```python
from build123d import *

# Parameters (mm, degrees)
F1_DEPTH  = 2
F2_R      = 2.5
F3_DEPTH  = 1.5
F4_R      = 1.3
F5_DEPTH  = 1.5
F7_DEPTH  = 7
F8_R      = 1.5
F9_DEPTH  = 10
F10_W     = 12.6
F10_H     = 2
F10_W_2   = 9.5
F11_DEPTH = 3.8
F12_R     = 3
F13_DEPTH = 0.4
F14_SIZE  = 1.49999
F15_W     = 19.2
F15_H     = 1.1
F16_DEPTH = 1


# Not quite as in the source:
# - a fillet or chamfer is up to 0.001 mm smaller than in the source, because OpenCascade refuses the exact size


with BuildPart() as f1:
    # F0 (on Top) → F1 (new body)
    with BuildSketch(Plane.XY):
        with BuildLine():
            Line((27.5, 38.5), (-27.5, 38.5))
            ThreePointArc((-27.5, 38.5), (-33.8639610307, 35.8639610307), (-36.5, 29.5))
            Line((-36.5, 29.5), (-36.5, -27.5))
            ThreePointArc((-36.5, -27.5), (-33.8639610307, -33.8639610307), (-27.5, -36.5))
            Line((-27.5, -36.5), (27.5, -36.5))
            ThreePointArc((27.5, -36.5), (33.8639610307, -33.8639610307), (36.5, -27.5))
            Line((36.5, -27.5), (36.5, 29.5))
            ThreePointArc((36.5, 29.5), (33.8639610307, 35.8639610307), (27.5, 38.5))
        make_face()
    extrude(amount=F1_DEPTH)

    # F2 (on face) → F3 (join)
    with BuildSketch(Plane.XY.offset(2)):
        with Locations((-19.24, -30.6)):
            Circle(F2_R)
        with Locations((8.96, -30.6)):
            Circle(F2_R)
        with Locations((24.16, 20.2)):
            Circle(F2_R)
        with Locations((-24.24, 21.5)):
            Circle(F2_R)
    extrude(amount=F3_DEPTH)

    # F4 (on face) → F5 (join)
    with BuildSketch(Plane.XY.offset(3.5)):
        with Locations((-19.24, -30.6)):
            Circle(F4_R)
        with Locations((8.96, -30.6)):
            Circle(F4_R)
        with Locations((24.16, 20.2)):
            Circle(F4_R)
        with Locations((-24.24, 21.5)):
            Circle(F4_R)
    extrude(amount=F5_DEPTH)

    # F6 (on face) → F7 (join)
    with BuildSketch(Plane.XY.offset(2)):
        with BuildLine():
            Line((27.5, 38.5), (-27.5, 38.5))
            ThreePointArc((-27.5, 38.5), (-33.8639610307, 35.8639610307), (-36.5, 29.5))
            Line((-36.5, 29.5), (-36.5, -27.5))
            ThreePointArc((-36.5, -27.5), (-33.8639610307, -33.8639610307), (-27.5, -36.5))
            Line((-27.5, -36.5), (27.5, -36.5))
            ThreePointArc((27.5, -36.5), (33.8639610307, -33.8639610307), (36.5, -27.5))
            Line((36.5, -27.5), (36.5, 29.5))
            ThreePointArc((36.5, 29.5), (33.8639610307, 35.8639610307), (27.5, 38.5))
        make_face()
        Polygon((-27.5, 29.5), (-27.5, 36.5), (27.5, 36.5), (27.5, 29.5), (34.5, 29.5), (34.5, -27.5), (27.5, -27.5), (27.5, -34.5), (-27.5, -34.5), (-27.5, -27.5), (-34.5, -27.5), (-34.5, 29.5), align=None, mode=Mode.SUBTRACT)
    extrude(amount=F7_DEPTH)

    # F8 (on face) → F9 (cut)
    with BuildSketch(Plane.XY.offset(9)):
        with Locations((-31, 33)):
            Circle(F8_R)
        with Locations((31, 33)):
            Circle(F8_R)
        with Locations((-31, -31)):
            Circle(F8_R)
        with Locations((31, -31)):
            Circle(F8_R)
    extrude(amount=-F9_DEPTH, mode=Mode.SUBTRACT)

    # F10 (on face) → F11 (cut)
    with BuildSketch(Plane.XY.offset(9)):
        with Locations((11.36, 37.5)):
            Rectangle(F10_W, F10_H)
        with Locations((-18.89, 37.5)):
            Rectangle(F10_W_2, F10_H)
    extrude(amount=-F11_DEPTH, mode=Mode.SUBTRACT)

    # F12 (on face) → F13 (cut)
    with BuildSketch(Plane(origin=(0, 0, 0), x_dir=(1, 0, 0), z_dir=(0, 0, -1))):
        with Locations((31, -33)):
            Circle(F12_R)
        with Locations((-31, -33)):
            Circle(F12_R)
        with Locations((-31, 31)):
            Circle(F12_R)
        with Locations((31, 31)):
            Circle(F12_R)
    extrude(amount=-F13_DEPTH, mode=Mode.SUBTRACT)

    # F14 (size 1.5 in the source; OpenCascade refuses exactly that, so slightly less here)
    f14_edges = [f1.edges().sort_by_distance(p)[0] for p in [
        (29.5, 33, 0.4),
        (-32.5, 33, 0.4),
        (29.5, -31, 0.4),
        (-32.5, -31, 0.4),
    ]]
    chamfer(f14_edges, length=F14_SIZE)

    # F15 (on face) → F16 (cut)
    with BuildSketch(Plane.XY.offset(9)):
        with BuildLine():
            Line((-23.64, 38.5), (-27.5, 38.5))
            ThreePointArc((-27.5, 38.5), (-33.8639610307, 35.8639610307), (-36.5, 29.5))
            Line((-36.5, 29.5), (-36.5, -27.5))
            ThreePointArc((-36.5, -27.5), (-33.8639610307, -33.8639610307), (-27.5, -36.5))
            Line((-27.5, -36.5), (27.5, -36.5))
            ThreePointArc((27.5, -36.5), (33.8639610307, -33.8639610307), (36.5, -27.5))
            Line((36.5, -27.5), (36.5, 29.5))
            ThreePointArc((36.5, 29.5), (33.8639610307, 35.8639610307), (27.5, 38.5))
            Line((27.5, 38.5), (17.66, 38.5))
            Line((17.66, 38.5), (17.66, 37.4))
            Line((17.66, 37.4), (27.5, 37.4))
            ThreePointArc((27.5, 37.4), (33.0861435714, 35.0861435714), (35.4, 29.5))
            Line((35.4, 29.5), (35.4, -27.5))
            ThreePointArc((35.4, -27.5), (33.0861435714, -33.0861435714), (27.5, -35.4))
            Line((27.5, -35.4), (-27.5, -35.4))
            ThreePointArc((-27.5, -35.4), (-33.0861435714, -33.0861435714), (-35.4, -27.5))
            Line((-35.4, -27.5), (-35.4, 29.5))
            ThreePointArc((-35.4, 29.5), (-33.0861435714, 35.0861435714), (-27.5, 37.4))
            Line((-27.5, 37.4), (-23.64, 37.4))
            Line((-23.64, 37.4), (-23.64, 38.5))
        make_face()
        with Locations((-4.54, 37.95)):
            Rectangle(F15_W, F15_H)
    extrude(amount=-F16_DEPTH, mode=Mode.SUBTRACT)


solid = f1.part
```
Here's how the part is built. I have some questions about the finished solid (model axes, mm). A direction names the side the tool comes from. Coordinates: 2 decimals unless noted, no trailing zeros. Order: outer loops, then holes, each group sorted by start corner. A loop starts at its lowest first (then second) coordinate and runs counter-clockwise, first axis right, second up.
1) Will these pins go through, and if not, where does the flat tip stop? pin 1 (4 mm diameter, centred on x = 25, y = 21, fed in from +Z); pin 2 (1 mm diameter, centred on x = 6, z = 7.5, fed in from +Y); pin 3 (0.5 mm diameter, centred on y = 3, z = 8.5, fed in from +X); pin 4 (1.1 mm diameter, centred on x = -6, z = 8.5, fed in from +Y).
2) Imagine slicing it at D-D on x = 8.96. List the corners of the cut face in (y, z) for me.
3) Imagine slicing it at C-C on y = -26. List the corners of the cut face in (x, z) for me, and give its area (3 significant figures).
4) I need wall thicknesses on line 1 (Y direction, x = -6.5, z = 6); line 2 (Y direction, x = -31, z = 4); line 3 (X direction, y = -2, z = 2.25). Which ranges of each line are inside material? Lowest first, please.
5) We'd pull the mould along Y, two halves only. Please class faces 1 (the face through (0, -34.5, 5)), 2 (the face through (-33.934, -33.794, 3.944)), 3 (the face through (11, 38, 5.2)): +Y half, -Y half, draft (parallel to the pull), parting line (faces both ways), or undercut.
6) Which directions (+Z, -Z, +X, -X, +Y, -Y) give clear straight access to the entire face, cutting with the end or side of a thin tool? Please do faces 4 (the face through (-18, -32, 3.5)), 5 (the face through (17.66, 37, 7)), 6 (the face through (-1, 2, 0)).
7) Imagine slicing it at A-A on x = 31. State how many separate pieces and enclosed holes the cut face has, and give its area (3 significant figures).
Response values:
1. pin 1: stops at z = 5
1. pin 2: stops at y = -34.5
1. pin 3: stops at x = 35.4
1. pin 4: stops at y = 38.5
2. outline: (-36.5, 0) - (38.5, 0) - (38.5, 5.2) - (36.5, 5.2) - (36.5, 2) - (-28.1, 2) - (-28.1, 3.5) - (-29.3, 3.5) - (-29.3, 5) - (-31.9, 5) - (-31.9, 3.5) - (-33.1, 3.5) - (-33.1, 2) - (-34.5, 2) - (-34.5, 9) - (-35.4, 9) - (-35.4, 8) - (-36.5, 8) - close
3. outline: (-36.5, 0) - (36.5, 0) - (36.5, 8) - (35.4, 8) - (35.4, 9) - (34.5, 9) - (34.5, 2) - (-34.5, 2) - (-34.5, 9) - (-35.4, 9) - (-35.4, 8) - (-36.5, 8) - close
3. area: 172 mm2
4. line 1: y = -36.5 to -34.5, 36.5 to 38.5
4. line 2: y = -35.79 to -32.5, -29.5 to -27.5, 29.5 to 31.5, 34.5 to 37.79
4. line 3: x = -36.5 to -34.5, 34.5 to 36.5
5. face 1: undercut
5. face 2: -Y half
5. face 3: draft
6. face 4: +Z
6. face 5: +Z, +Y
6. face 6: -Z, +X, -X, +Y, -Y
7. separate pieces: 3
7. enclosed holes: 0
7. area: 200 mm2
